Check sheet for the modelled part. Datum: model origin and axes. Units: mm. Round coordinates to 2 decimals unless told otherwise and drop trailing zeros. Order: outer loops, then holes, each group sorted by start corner. A loop starts at its lowest first (then second) coordinate and runs counter-clockwise, first axis right, second up.
Q1. Scan lines: probe 1 along X at (y, z) = (0.95, -1.75); probe 2 along Z at (x, y) = (4, 0.55). Record each from-to range of solid material in increasing order.
Q2. Cross-section at A-A on x = 4. Record the cut outline in (y, z), then the cut area to 3 significant figures.
Q3. Cross-section at B-B on y = 0.8. Record the cut outline in (x, z).
Q4. Depth check by flat-ended pin: P1, Ø3, axis at x = 29, z = -20.5, coming from the -Y side. Enter the tip coordinate at first touch or a pass-through.
from build123d import *

# Parameters (mm, degrees)
SKETCH1_W           = 40
SKETCH1_H           = 24
BOSS_EXTRUDE1_DEPTH = 2
SKETCH2_W           = 40
SKETCH2_H           = 24
SKETCH2_W_2         = 36
SKETCH2_H_2         = 22
BOSS_EXTRUDE3_DEPTH = 8
SKETCH5_W           = 4
SKETCH5_H           = 3
CUT_EXTRUDE1_DEPTH  = 2
SKETCH6_W           = 24
SKETCH6_H           = 10
CUT_EXTRUDE2_DEPTH  = 2
SKETCH7_W           = 22
SKETCH7_H           = 8
CUT_EXTRUDE3_DEPTH  = 2
SKETCH8_W           = 1
SKETCH8_H           = 3
CUT_EXTRUDE4_DEPTH  = 2
SKETCH9_W           = 38
SKETCH9_H           = 24
CUT_EXTRUDE5_DEPTH  = 9


with BuildPart() as part:
    # Sketch1 → Boss-Extrude1 (new body)
    with BuildSketch(Plane(origin=(0, 0, 0), x_dir=(1, 0, 0), z_dir=(0, 1, 0))):
        with Locations((20, 12)):
            Rectangle(SKETCH1_W, SKETCH1_H)
    extrude(amount=BOSS_EXTRUDE1_DEPTH)

    # Sketch2 → Boss-Extrude3 (add)
    with BuildSketch(Plane(origin=(0, 2, 0), x_dir=(1, 0, 0), z_dir=(0, 1, 0))):
        with Locations((20, 12)):
            Rectangle(SKETCH2_W, SKETCH2_H)
        with Locations((21, 12)):
            Rectangle(SKETCH2_W_2, SKETCH2_H_2, mode=Mode.SUBTRACT)
    extrude(amount=BOSS_EXTRUDE3_DEPTH)

    # Sketch5 → Cut-Extrude1 (cut)
    with BuildSketch(Plane(origin=(0, 2, 0), x_dir=(1, 0, 0), z_dir=(0, 1, 0))):
        with Locations((6, 2.5)):
            Rectangle(SKETCH5_W, SKETCH5_H)
    extrude(amount=-CUT_EXTRUDE1_DEPTH, mode=Mode.SUBTRACT)

    # Sketch6 → Cut-Extrude2 (cut)
    with BuildSketch(Plane(origin=(40, 0, 0), x_dir=(0, 0, -1), z_dir=(1, 0, 0))):
        with Locations((12, 5)):
            Rectangle(SKETCH6_W, SKETCH6_H)
    extrude(amount=-CUT_EXTRUDE2_DEPTH, mode=Mode.SUBTRACT)

    # Sketch7 → Cut-Extrude3 (cut)
    with BuildSketch(Plane(origin=(3, 0, 0), x_dir=(0, 0, -1), z_dir=(1, 0, 0))):
        with Locations((12, 6)):
            Rectangle(SKETCH7_W, SKETCH7_H)
    extrude(amount=-CUT_EXTRUDE3_DEPTH, mode=Mode.SUBTRACT)

    # Sketch8 → Cut-Extrude4 (cut)
    with BuildSketch(Plane(origin=(0, 2, 0), x_dir=(1, 0, 0), z_dir=(0, 1, 0))):
        with Locations((3.5, 2.5)):
            Rectangle(SKETCH8_W, SKETCH8_H)
    extrude(amount=-CUT_EXTRUDE4_DEPTH, mode=Mode.SUBTRACT)

    # Sketch9 → Cut-Extrude5 (cut)
    with BuildSketch(Plane(origin=(0, 10, 0), x_dir=(1, 0, 0), z_dir=(0, 1, 0))):
        with Locations((19, 12)):
            Rectangle(SKETCH9_W, SKETCH9_H)
    extrude(amount=-CUT_EXTRUDE5_DEPTH, mode=Mode.SUBTRACT)


solid = part.part
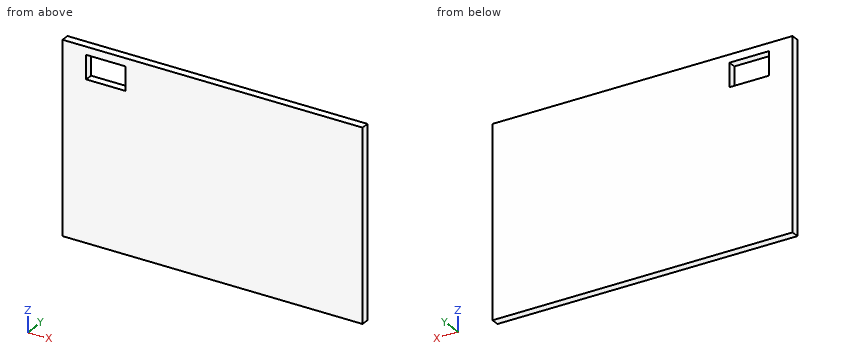
Results found:
1. probe 1: x = 0 to 3, 8 to 38
1. probe 2: z = -24 to -4, -1 to 0
2. outline: (0, -24) - (1, -24) - (1, -4) - (0, -4) - close; (0, -1) - (1, -1) - (1, 0) - (0, 0) - close
2. area: 21.0 mm2
3. outline: (0, -24) - (38, -24) - (38, 0) - (0, 0) - close; hole (3, -4) - (8, -4) - (8, -1) - (3, -1) - close
4. P1: stops at y = 0
